from build123d import *

# Parameters (mm, degrees)
EXTRUDE_1_DEPTH = 10
SKETCH_2_W      = 35
SKETCH_2_H      = 4
EXTRUDE_2_DEPTH = 100


with BuildPart() as part:
    # 草图1 → 凸台-拉伸1 (new body)
    with BuildSketch(Plane.XY):
        with BuildLine():
            Line((-17.5, 0), (-17.5, -25))
            Line((-17.5, -25), (17.5, -25))
            Line((17.5, -25), (17.5, 0))
            ThreePointArc((17.5, 0), (0, 17.5), (-17.5, 0))
        make_face()
    extrude(amount=EXTRUDE_1_DEPTH)

    # 草图2 → 凸台-拉伸2 (add)
    with BuildSketch(Plane.XY.offset(10)):
        with Locations((0, -23)):
            Rectangle(SKETCH_2_W, SKETCH_2_H)
    extrude(amount=EXTRUDE_2_DEPTH)


solid = part.part
Verification items for the finished model (mm, model axes). A direction names the side the tool comes from. Give positions to 0.01 mm unless a question says otherwise; leave off trailing zeros. Write each loop counter-clockwise with the first axis right and the second up, starting at its lowest first coordinate (ties: lowest second). Pieces come first, ordered by that corner, then holes.
(1) Cross-section at C-C (z = 14). Enter the section's corners in (x, y), plus the area to 3 significant figures.
(2) Cross-section at A-A (x = 0). Enter the section's corners in (y, z), plus the area to 3 significant figures.
(3) Cross-section at B-B (y = -12). Enter the section's corners in (x, z), plus the area to 3 significant figures.
(4) Gauge pin test, flat ends, axial feed: pin 1 (4 mm diameter, centred on x = -1, z = 14.5, fed in from +Y); pin 2 (6 mm diameter, centred on x = 4.5, y = 9.5, fed in from +Z). Record the tip position at first contact, or that the pin passes through.
(5) Cross-section at D-D (x = -11.5). Enter the section's corners in (y, z).
(6) Access from +Z, -Z, +X, -X, +Y, -Y to the whole of each face (thin tool, end or side, straight path). Record for faces 1 (the face through (0, -23, 110)), 2 (the face through (0, -21, 59)).
(7) Material ranges on line 1 (Z direction, x = 7.5, y = 8); line 2 (Y direction, x = 3.5, z = 44.5), recorded low to high.
Worked out:
1. outline: (-17.5, -25) - (17.5, -25) - (17.5, -21) - (-17.5, -21) - close
1. area: 140 mm2
2. outline: (-25, 0) - (17.5, 0) - (17.5, 10) - (-21, 10) - (-21, 110) - (-25, 110) - close
2. area: 825 mm2
3. outline: (-17.5, 0) - (17.5, 0) - (17.5, 10) - (-17.5, 10) - close
3. area: 350 mm2
4. pin 1: stops at y = -21
4. pin 2: stops at z = 10
5. outline: (-25, 0) - (13.19, 0) - (13.19, 10) - (-21, 10) - (-21, 110) - (-25, 110) - close
6. face 1: +Z, +X, -X, +Y, -Y
6. face 2: +Z, +X, -X, +Y
7. line 1: z = 0 to 10
7. line 2: y = -25 to -21
